Solid Edge part; units mm, degrees
sketch "Sketch1" plane through (0, 0, 0) normal (0, -1, 0) x (1, 0, 0)
  line L0 (11, 5) -> (16.5, 5)
  line L1 (16.5, 5) -> (16.5, 250)
  line L2 (16.5, 250) -> (37.1963, 250)
  line L3 (37.1963, 250) -> (37.1963, 256)
  line L4 (27, 256) -> (37.1963, 256)
  line L5 (27, 260) -> (27, 256)
  line L6 (16, 260) -> (27, 260)
  line L7 (16, 256) -> (16, 260)
  line L8 (11, 256) -> (16, 256)
  line L9 (11, 5) -> (11, 256)
  dimension "D1" = 37.1963
  dimension "D2" = 27
  dimension "D3" = 16
revolve "RevolvedProtrusion1" add sketch "Sketch1" angle 360 about axis through (0, 0, 0) along (0, 0, 1)
hole "Hole1" at (0, 0, 19) direction (-1, 0, 0) diameter 4.134 end through all
hole "Hole_2" at (0, 0, 19) direction (1, 0, 0) diameter 5.5 end up to next
hole "Hole_3" at (32, 0, 256) direction (0, 0, -1) diameter 4.134 end through all
pattern_circular "Pattern1" count 6 over 360 about axis through (0, 0, 260) along (0, 0, -1) of "Hole_3"
chamfer "Chamfer_1" distance 0.5 angle 45 7 edges at (-11, 0, 5) (-16.5, 0, 5) (-37.1963, 0, 250) (-37.1963, 0, 256) (-27, 0, 260) (-16, 0, 260) (-11, 0, 256)
pattern_circular "Pattern3" count 3 over 360 about axis through (0, 0, 5) along (0, 0, 1) of "Hole_2", "Hole1"
properties material "Steel"
The model under review builds one solid part; all positions refer to its coordinate system, in mm. A direction names the side the tool comes from. Round coordinates to 2 decimals unless told otherwise and drop trailing zeros. Answer in a Markdown table with one row per item.
1) Draft analysis for pull direction Z (two halves, no side actions). For faces 1 (the flat face through (-11, 4, 256)), 2 (the cylindrical face through (-5.85, 26.36, 257.73)), 3 (the cylindrical face through (-6.872, 11.661, 16.253)), state which applies: pulls with the +Z half, pulls with the -Z half, needs draft (parallel to the pull), parting line crosses it, or undercut.
Taken from the geometry:
| item | result |
|---|---|
| face 1 | pulls with the +Z half |
| face 2 | needs draft |
| face 3 | undercut |
2) Tool access review of faces 4 (the cylindrical face through (35.48, 11.17, 253.04)), 5 (the cylindrical face through (-6.663, -11.782, 16.253)), 6 (the flat face through (16, -8, 250)), 7 (the cylindrical face through (-3.47, -15.62, 257.77)), 8 (the cylindrical face through (13.534, 0.121, 16.253)): name each direction out of +Z, -Z, +X, -X, +Y, -Y from which nothing blocks a thin tool from reaching the whole face with its end or side.
Taken from the geometry:
| item | result |
|---|---|
| face 4 | +Z, -Z |
| face 5 | none |
| face 6 | -Z |
| face 7 | +Z |
| face 8 | +X |
3) Wall thickness on line 1 along X through (y, z) = (0, 84.5); line 2 along Y through (x, z) = (0, 258): over which ranges is each line inside the solid? List them lowest first.
Taken from the geometry:
| item | result |
|---|---|
| line 1 | x = -16.5 to -11, 11 to 16.5 |
| line 2 | y = -27 to -16, 16 to 27 |
4) For pin 1 Ø5 at (y, z) = (0, 19) entering from -X; pin 2 Ø8 at (x, y) = (20.5, 26) entering from -Z; pin 3 Ø3.5 at (x, y) = (32, 0) entering from +Z; pin 4 Ø6 at (x, z) = (5, 198.5) entering from +Y, all flat-tipped, find the tip position at first contact; note any pin that passes through.
Taken from the geometry:
| item | result |
|---|---|
| pin 1 | stops at x = -16.5 |
| pin 2 | stops at z = 250 |
| pin 3 | passes through |
| pin 4 | stops at y = 16.38 |
